from build123d import *

# Parameters (mm, degrees)
F0_W      = 62
F0_H      = 35
F1_DEPTH  = 5
F2_R      = 1.5
F3_DEPTH  = 5
F4_R      = 3
F5_DEPTH  = 3.5
F6_R      = 3
F7_DEPTH  = 3.5
F8_R      = 1.5
F9_DEPTH  = 5
F10_R     = 1.5
F11_DEPTH = 5
F12_R     = 3
F13_DEPTH = 3.5


with BuildPart() as f1:
    # F0 (on Top) → F1 (new body)
    with BuildSketch(Plane.XY):
        Rectangle(F0_W, F0_H)
    extrude(amount=F1_DEPTH)

    # F2 (on face) → F3 (cut)
    with BuildSketch(Plane.XY.offset(5)):
        with Locations((-28.5, 7.5)):
            Circle(F2_R)
        with Locations((-21, 15)):
            Circle(F2_R)
    extrude(amount=-F3_DEPTH, mode=Mode.SUBTRACT)

    # F4 (on face) → F5 (cut)
    with BuildSketch(Plane(origin=(0, 0, 0), x_dir=(1, 0, 0), z_dir=(0, 0, -1))):
        with Locations((-28.5, -7.5)):
            Circle(F4_R)
        with Locations((-21, -15)):
            Circle(F4_R)
    extrude(amount=-F5_DEPTH, mode=Mode.SUBTRACT)

    # F6 (on face) → F7 (cut)
    with BuildSketch(Plane.XY.offset(5)):
        with Locations((-16, 2.5)):
            Circle(F6_R)
    extrude(amount=-F7_DEPTH, mode=Mode.SUBTRACT)

    # F8 (on face) → F9 (cut)
    with BuildSketch(Plane.XY.offset(1.5)):
        with Locations((-16, 2.5)):
            Circle(F8_R)
    extrude(amount=-F9_DEPTH, mode=Mode.SUBTRACT)

    # F10 (on face) → F11 (cut)
    with BuildSketch(Plane.XY.offset(5)):
        with Locations((16, 10.5)):
            Circle(F10_R)
        with Locations((16, -14)):
            Circle(F10_R)
    extrude(amount=-F11_DEPTH, mode=Mode.SUBTRACT)

    # F12 (on face) → F13 (cut)
    with BuildSketch(Plane(origin=(0, 0, 0), x_dir=(1, 0, 0), z_dir=(0, 0, -1))):
        with Locations((16, 14)):
            Circle(F12_R)
        with Locations((16, -10.5)):
            Circle(F12_R)
    extrude(amount=-F13_DEPTH, mode=Mode.SUBTRACT)


solid = f1.part
The model under review builds one solid part; all positions refer to its coordinate system, in mm. A direction names the side the tool comes from. Round coordinates to 2 decimals unless told otherwise and drop trailing zeros. Write each loop counter-clockwise with the first axis right and the second up, starting at its lowest first coordinate (ties: lowest second). Pieces come first, ordered by that corner, then holes. Notation, with made-up numbers: M -29.5,-0.75 L -6.5,-0.75 A21 cw -6.5,7.25 Z; hole C 41,74 d5. An arc over 180 degrees is marked long. Use a Markdown table: item, result. Add a question column.
Q1. We need section C-C, the plane x = -21. State the section outline as (y, z) points, plus the area to 3 significant figures.
Q2. We need section D-D, the plane z = 2.15. State the section outline as (x, y) points.
Q3. To check wall thickness, follow line 1 (Y direction, x = 16, z = 1.15); line 2 (X direction, y = 15, z = 0.45); line 3 (Y direction, x = -28.5, z = 4.45). State the ranges of each line that lie inside material, in increasing order.
Q4. Machinability: for faces 4 (the face through (-21, 12, 2)), 5 (the face through (-19, 2.6, 3.3)), 6 (the face through (14.5, 10.57, 4.26)), which of the approach directions +Z, -Z, +X, -X, +Y, -Y give a long, thin tool a straight path to every point of the face, cutting with its end or side? Answer none if there is none.
Q5. The part is to be moulded in two halves that separate along X. For faces 1 (the face through (0, -17.5, 2)), 2 (the face through (-31, 0, 2)), 3 (the face through (-22.5, 15.07, 4.26)), say which applies: pulls with the +X half, pulls with the -X half, needs draft (parallel to the pull), parting line crosses it, or undercut.
Q6. We need section B-B, the plane y = 2.5. State the section outline as (x, z) points.
Q7. Insertion check: pin 1 (1.8 mm diameter, centred on x = 16, y = -14, fed in from +Z); pin 2 (1.6 mm diameter, centred on x = -22.5, y = 15, fed in from -Z); pin 3 (3 mm diameter, centred on x = -16.5, y = 3.5, fed in from +Z). Each pin has a flat end and moves straight along its axis. Give the tip position at first contact, or say it passes through.
Q8. We need section A-A, the plane x = 16. State the section outline as (y, z) points.
Findings below:
| question | item | result |
|---|---|---|
| 1 | outline | M -17.5,0 L 12,0 L 12,3.5 L 13.5,3.5 L 13.5,5 L -17.5,5 Z; M 16.5,3.5 L 17.5,3.5 L 17.5,5 L 16.5,5 Z |
| 1 | area | 151 mm² |
| 2 | outline | M -31,-17.5 L 31,-17.5 L 31,17.5 L -19.34,17.5 A3 cw long -22.66,17.5 L -31,17.5 L -31,9.16 A3 cw long -31,5.84 Z; hole C -16,2.5 d6; hole C 16,-14 d6; hole C 16,10.5 d6 |
| 3 | line 1 | y = -17.5 to -17, -11 to 7.5, 13.5 to 17.5 |
| 3 | line 2 | x = -31 to -24, -18 to 31 |
| 3 | line 3 | y = -17.5 to 6, 9 to 17.5 |
| 4 | face 4 | -Z |
| 4 | face 5 | +Z |
| 4 | face 6 | +Z, -Z |
| 5 | face 1 | needs draft |
| 5 | face 2 | pulls with the -X half |
| 5 | face 3 | undercut |
| 6 | outline | M -31,0 L -17.5,0 L -17.5,1.5 L -19,1.5 L -19,5 L -31,5 Z; M -14.5,0 L 31,0 L 31,5 L -13,5 L -13,1.5 L -14.5,1.5 Z |
| 7 | pin 1 | passes through |
| 7 | pin 2 | stops at z = 3.5 |
| 7 | pin 3 | stops at z = 1.5 |
| 8 | outline | M -17.5,0 L -17,0 L -17,3.5 L -15.5,3.5 L -15.5,5 L -17.5,5 Z; M -12.5,3.5 L -11,3.5 L -11,0 L 7.5,0 L 7.5,3.5 L 9,3.5 L 9,5 L -12.5,5 Z; M 12,3.5 L 13.5,3.5 L 13.5,0 L 17.5,0 L 17.5,5 L 12,5 Z |
